from build123d import *

# Parameters (mm, degrees)
F0_W     = 1.8361258607
F0_H     = 1.0668
F0_W_2   = 7.62
F0_H_2   = 160.4273358566
F1_DEPTH = 10.16
F2_DEPTH = 5.08


with BuildPart() as f1:
    # F0 (on Top) → F1 (new body)
    with BuildSketch(Plane.XY):
        Polygon((6.7189444143, 102.6402935386), (6.7189444143, 103.7061576819), (-2.1710555857, 103.7061576819), (-11.0610555857, 103.7061576819), (-11.0610555857, 102.6402935386), (-5.9810555857, 102.6402935386), (1.6389444143, 102.6402935386), align=None)
        with BuildLine():
            Line((-2.1710555857, 103.7061576819), (6.7189444143, 103.7061576819))
            Line((6.7189444143, 103.7061576819), (10.3688539856, 118.139948899))
            ThreePointArc((10.3688539856, 118.139948899), (5.2686232822, 112.2832362473), (-2.1710555857, 110.0550947226))
            Line((-2.1710555857, 110.0550947226), (-2.1710555857, 103.7061576819))
        make_face()
        with BuildLine():
            Line((-11.0610555857, 103.7061576819), (-2.1710555857, 103.7061576819))
            Line((-2.1710555857, 103.7061576819), (-2.1710555857, 110.0550947226))
            ThreePointArc((-2.1710555857, 110.0550947226), (-9.3601607133, 111.9690507219), (-14.5474187039, 117.301856235))
            Line((-14.5474187039, 117.301856235), (-11.0610555857, 103.7061576819))
        make_face()
        with BuildLine():
            ThreePointArc((-2.1710555857, 110.0550947226), (5.2686232822, 112.2832362473), (10.3688539856, 118.139948899))
            Line((10.3688539856, 118.139948899), (11.6430755059, 123.1789360379))
            ThreePointArc((11.6430755059, 123.1789360379), (11.6622834114, 123.6015178338), (11.668688004, 124.0244874534))
            Line((11.668688004, 124.0244874534), (2.778688004, 124.0244874534))
            ThreePointArc((2.778688004, 124.0244874534), (1.3365515641, 120.4787366559), (-2.1710555857, 118.9461576819))
            Line((-2.1710555857, 118.9461576819), (-2.1710555857, 110.0550947226))
        make_face()
        with Locations((5.8008814839, -58.3204423181)):
            Rectangle(F0_W, F0_H)
        with Locations((-2.1710555857, 22.4266256103)):
            Rectangle(F0_W_2, F0_H_2)
        with BuildLine():
            ThreePointArc((-14.5474187039, 117.301856235), (-9.3601607133, 111.9690507219), (-2.1710555857, 110.0550947226))
            Line((-2.1710555857, 110.0550947226), (-2.1710555857, 118.9461576819))
            ThreePointArc((-2.1710555857, 118.9461576819), (-5.8470627935, 120.3866238933), (-7.381311996, 124.0244874534))
            Line((-7.381311996, 124.0244874534), (-16.271311996, 124.0244874534))
            Line((-16.271311996, 124.0244874534), (-14.5474187039, 117.301856235))
        make_face()
        with BuildLine():
            Line((10.1554150025, -72.599724671), (6.7189444143, -58.8538423181))
            Line((6.7189444143, -58.8538423181), (4.8828185536, -58.8538423181))
            Line((4.8828185536, -58.8538423181), (-2.1710555857, -58.8538423181))
            Line((-2.1710555857, -58.8538423181), (-2.1710555857, -65.2038423181))
            ThreePointArc((-2.1710555857, -65.2038423181), (5.0164501176, -67.1946661459), (10.1554150025, -72.599724671))
        make_face()
        Polygon((4.8828185536, -58.8538423181), (4.8828185536, -57.7870423181), (1.6389444143, -57.7870423181), (-5.9810555857, -57.7870423181), (-11.0610555857, -57.7870423181), (-11.0610555857, -58.8538423181), (-2.1710555857, -58.8538423181), align=None)
        with BuildLine():
            Line((2.778688004, 124.0244874534), (11.668688004, 124.0244874534))
            ThreePointArc((11.668688004, 124.0244874534), (-2.301311996, 137.9944874534), (-16.271311996, 124.0244874534))
            Line((-16.271311996, 124.0244874534), (-7.381311996, 124.0244874534))
            ThreePointArc((-7.381311996, 124.0244874534), (-5.9391755561, 127.5702382509), (-2.4315684063, 129.1028172248))
            ThreePointArc((-2.4315684063, 129.1028172248), (1.2444388015, 127.6623510135), (2.778688004, 124.0244874534))
        make_face()
        with BuildLine():
            Line((11.7989444143, -79.1738423181), (10.1554150025, -72.599724671))
            ThreePointArc((10.1554150025, -72.599724671), (5.0164501176, -67.1946661459), (-2.1710555857, -65.2038423181))
            ThreePointArc((-2.1710555857, -65.2038423181), (-9.3585612891, -67.1946661459), (-14.497526174, -72.599724671))
            Line((-14.497526174, -72.599724671), (-16.1410555857, -79.1738423181))
            ThreePointArc((-16.1410555857, -79.1738423181), (-2.1710555857, -93.1438423181), (11.7989444143, -79.1738423181))
        make_face()
        with BuildLine():
            ThreePointArc((2.9089444143, -79.1738423181), (-5.7631580342, -82.7659447665), (-2.1710555857, -74.0938423181))
            ThreePointArc((-2.1710555857, -74.0938423181), (1.4210468627, -75.5817398696), (2.9089444143, -79.1738423181))
        make_face(mode=Mode.SUBTRACT)
        with BuildLine():
            Line((-2.1710555857, -65.2038423181), (-2.1710555857, -58.8538423181))
            Line((-2.1710555857, -58.8538423181), (-11.0610555857, -58.8538423181))
            Line((-11.0610555857, -58.8538423181), (-14.497526174, -72.599724671))
            ThreePointArc((-14.497526174, -72.599724671), (-9.3585612891, -67.1946661459), (-2.1710555857, -65.2038423181))
        make_face()
    extrude(amount=F1_DEPTH)

    # F2 (add): a face of the model
    f2_faces = [f1.faces().sort_by_distance(p)[0] for p in [
        (1.6389444143, 22.4266256103, 5.08),
    ]]
    extrude(f2_faces, amount=F2_DEPTH)


solid = f1.part
For this review, take the finished solid that the model builds, in its own axes (mm). A direction names the side the tool comes from. Give positions to 0.01 mm unless a question says otherwise; leave off trailing zeros. Loops run counter-clockwise (first coordinate to the right, second up) from the corner with the lowest first, then second, coordinate; pieces in that order, holes last. Notation, with made-up numbers: M 44,-10.75 L 81,-10.75 A38 cw 81,28.25 Z; hole C -9.75,13 d7. An arc over 180 degrees is marked long. Answer as a JSON object with one key per item and string values. Group by question number.
Q1. Add section B-B on y = -23. Give the boundary of the cut face in (x, z).
Q2. Tool access review of faces 5 (the flat face through (6.719, 21, 5)), 6 (the flat face through (-13.7, 114, 5)), 7 (the flat face through (-2, 21, 10.16)): name each direction out of +Z, -Z, +X, -X, +Y, -Y from which nothing blocks a thin tool from reaching the whole face with its end or side.
Q3. Add section A-A on z = 7. Give the boundary of the cut face in (x, y).
Q4. Insertion check: P1, Ø1.2, axis at y = -58.5, z = 3, coming from the -X side; P2, Ø5, axis at y = 33, z = 5.5, coming from the +X side; P3, Ø2.5, axis at x = -7.5, z = 7, coming from the -Y side; P4, Ø6, axis at x = -2.17, y = -79.17, coming from the +Z side. Each pin has a flat end and moves straight along its axis. Give the tip position at first contact, or say it passes through.
Q5. Mouldability with a two-part tool opening along Y and no side actions: class faces 1 (the flat face through (-8, -57.787, 5)), 2 (the flat face through (-2, 21, 0)), 3 (the cylindrical face through (-2.48, -93.14, 5.01)), 4 (the flat face through (-5.981, 21, 5)) as +Y half, -Y half, draft (parallel to the pull), parting line (faces both ways), or undercut.
Q6. For probe 1 along Y at (x, z) = (-5, 4.75); probe 2 along Y at (x, z) = (-5.25, 6.75); probe 3 along X at (y, z) = (-35.5, 5.75), list the stretches that pass through material, from the lowest coordinate up. Write a range as [from, to].
Checked values:
{
 "1": {"outline": "M -5.98,0 L 6.72,0 L 6.72,10.16 L -5.98,10.16 Z"},
 "2": {"face 5": "+Z, -Z, +X", "face 6": "+Z, -Z, -X", "face 7": "+Z, +X, -X, +Y, -Y"},
 "3": {"outline": "M -16.27,124.02 L -11.06,103.71 L -11.06,102.64 L -5.98,102.64 L -5.98,-57.79 L -11.06,-57.79 L -11.06,-58.85 L -16.14,-79.17 A13.97 ccw 11.8,-79.17 L 6.72,-58.85 L 6.72,103.71 L 11.64,123.18 A13.97 ccw long Z; hole C -2.3,124.02 d10.16; hole C -2.17,-79.17 d10.16"},
 "4": {"P1": "x = -11.12", "P2": "x = 6.72", "P3": "y = -92.54", "P4": "through"},
 "5": {"face 1": "undercut", "face 2": "draft", "face 3": "-Y half", "face 4": "undercut"},
 "6": {"probe 1": "[-92.85, -83.39], [-74.95, 119.72], [128.33, 137.73]", "probe 2": "[-92.8, -83.21], [-75.13, 119.89], [128.16, 137.68]", "probe 3": "[-5.98, 6.72]"}
}
